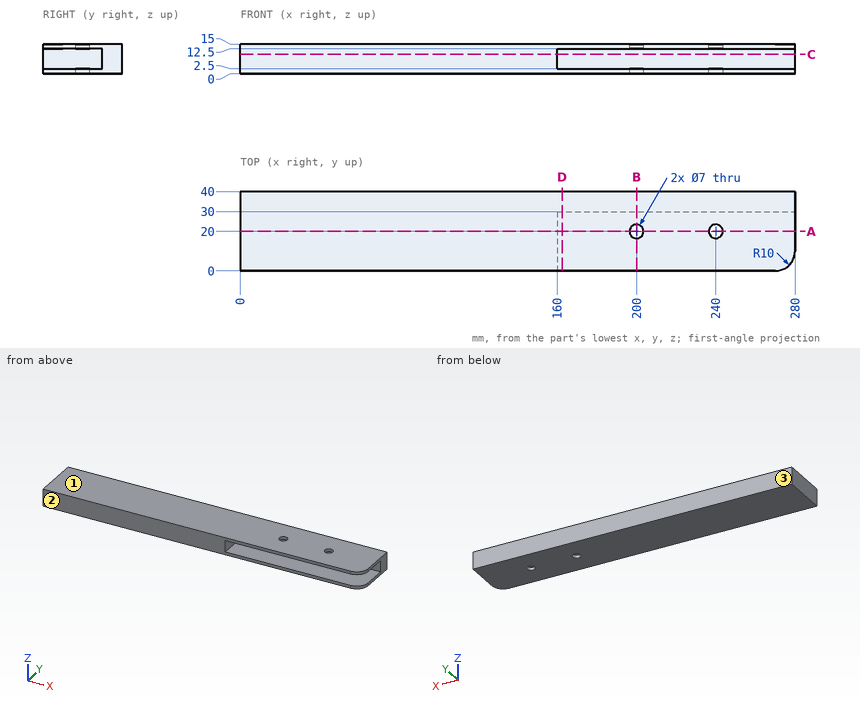
Verification items for this drawing (mm, ordinates from the low corner). Give positions to 0.01 mm unless a question says otherwise; leave off trailing zeros. Order: outer loops, then holes, each group sorted by start corner. A loop starts at its lowest first (then second) coordinate and runs counter-clockwise, first axis right, second up. Notation, with made-up numbers: M 3,-34 L 24,-34 A14 cw 24,-26 Z; hole C 69.5,4 d7. An arc over 180 degrees is marked long. Use a Markdown table: item, result.
Item 1: Section check C-C (z = 9.75). Record the cut outline in (x, y), and give its area (3 significant figures).
Answers follow:
| item | result |
|---|---|
| outline | M 0,0 L 160,0 L 160,30 L 280,30 L 280,40 L 0,40 Z |
| area | 7,600 mm2 |
Item 2: Section check A-A (y = 20). Record the cut outline in (x, z), and give its area (3 significant figures).
Answers follow:
| item | result |
|---|---|
| outline | M 0,0 L 196.5,0 L 196.5,2.5 L 160,2.5 L 160,12.5 L 196.5,12.5 L 196.5,15 L 0,15 Z; M 203.5,0 L 236.5,0 L 236.5,2.5 L 203.5,2.5 Z; M 203.5,12.5 L 236.5,12.5 L 236.5,15 L 203.5,15 Z; M 243.5,0 L 280,0 L 280,2.5 L 243.5,2.5 Z; M 243.5,12.5 L 280,12.5 L 280,15 L 243.5,15 Z |
| area | 2,930 mm2 |
Item 3: Draft check along Y on the marked faces 1, 2 and 3. Enter one of: +Y half, -Y half, draft (parallel to the pull), parting line (faces both ways), or undercut.
Answers follow:
| item | result |
|---|---|
| face 1 | draft |
| face 2 | -Y half |
| face 3 | +Y half |
Item 4: Section check D-D (x = 162.5). Record the cut outline in (y, z), and give its area (3 significant figures).
Answers follow:
| item | result |
|---|---|
| outline | M 0,0 L 40,0 L 40,15 L 0,15 L 0,12.5 L 30,12.5 L 30,2.5 L 0,2.5 Z |
| area | 300 mm2 |
Item 5: Section check B-B (x = 200). Record the cut outline in (y, z).
Answers follow:
| item | result |
|---|---|
| outline | M 0,0 L 16.5,0 L 16.5,2.5 L 0,2.5 Z; M 0,12.5 L 16.5,12.5 L 16.5,15 L 0,15 Z; M 23.5,0 L 40,0 L 40,15 L 23.5,15 L 23.5,12.5 L 30,12.5 L 30,2.5 L 23.5,2.5 Z |
Item 6: Depth check by flat-ended pin: P1, Ø5, axis at x = 246, z = 8, coming from the -Y side; P2, Ø8, axis at x = 230.5, y = 9.5, coming from the -Z side; P3, Ø3, axis at y = 15, z = 5.5, coming from the +X side. Enter the tip coordinate at first touch or a pass-through.
Answers follow:
| item | result |
|---|---|
| P1 | stops at y = 30 |
| P2 | stops at z = 0 |
| P3 | stops at x = 160 |
Item 7: Material ranges on line 1 along Y through (x, z) = (240, 1); line 2 along Z through (x, y) = (261, 23.5); line 3 along X through (y, z) = (9, 7.75), recorded low to high.
Answers follow:
| item | result |
|---|---|
| line 1 | y = 0 to 16.5, 23.5 to 40 |
| line 2 | z = 0 to 2.5, 12.5 to 15 |
| line 3 | x = 0 to 160 |
